```python
from build123d import *

# Parameters (mm, degrees)
ESBO_O1_W                = 86.5
ESBO_O1_H                = 54.64
RESSALTO_EXTRUS_O2_DEPTH = 2
ESBO_O3_R                = 1.59
CORTE_EXTRUS_O1_DEPTH    = 2
FILETE1_R                = 12
FILETE2_R                = 12
ESBO_O4_R                = 5
ESBO_O4_R_2              = 4
ESBO_O4_W                = 6
ESBO_O4_H                = 8.5
CORTE_EXTRUS_O2_DEPTH    = 10


with BuildPart() as part:
    # Esboço1 → Ressalto-extrusão2 (new body)
    with BuildSketch(Plane.XY):
        with Locations((43.25, 27.32)):
            Rectangle(ESBO_O1_W, ESBO_O1_H)
    extrude(amount=RESSALTO_EXTRUS_O2_DEPTH)

    # Esboço3 → Corte-extrusão1 (cut)
    with BuildSketch(Plane(origin=(0, 0, 0), x_dir=(-1, 0, 0), z_dir=(0, 0, -1))):
        with Locations((-71.89, 51.46)):
            Circle(ESBO_O3_R)
        with Locations((-71.89, 3.18)):
            Circle(ESBO_O3_R)
        with Locations((-5.72, 6.35)):
            Circle(ESBO_O3_R)
        with Locations((-5.72, 48.29)):
            Circle(ESBO_O3_R)
    extrude(amount=-CORTE_EXTRUS_O1_DEPTH, mode=Mode.SUBTRACT)

    # Filete1
    filete1_edges = [part.edges().sort_by_distance(p)[0] for p in [
        (0, 54.64, 1),
    ]]
    fillet(filete1_edges, radius=FILETE1_R)

    # Filete2
    filete2_edges = [part.edges().sort_by_distance(p)[0] for p in [
        (0, 0, 1),
    ]]
    fillet(filete2_edges, radius=FILETE2_R)

    # Esboço4 → Corte-extrusão2 (cut)
    with BuildSketch(Plane.XY.offset(2)):
        with Locations((24.86, 48.58)):
            Circle(ESBO_O4_R)
        with Locations((39.09, 49.5)):
            Circle(ESBO_O4_R_2)
        with Locations((64.16, 46.97)):
            Circle(ESBO_O4_R_2)
        with Locations((83.5, 38.39)):
            Rectangle(ESBO_O4_W, ESBO_O4_H)
    extrude(amount=-CORTE_EXTRUS_O2_DEPTH, mode=Mode.SUBTRACT)


solid = part.part
```
Source: CAD feature listing. Evaluate the final solid. Frame: model axes, mm. A direction names the side the tool comes from. Coordinates: 2 decimals unless noted, no trailing zeros. Write each loop counter-clockwise with the first axis right and the second up, starting at its lowest first coordinate (ties: lowest second). Pieces come first, ordered by that corner, then holes. Notation, with made-up numbers: (3, -16.5) -> (23, -16.5) arc R36 cw to (23, 22.5) -> close; hole circle Ø1 at (73.5, 60.5). An arc over 180 degrees is marked (long way). Return JSON: item names as keys, results as strings. Group by question number.
1) Contact query for a flat-ended pin moving along its axis: P1, Ø5, axis at x = 64.16, y = 46.97, coming from the -Z side. Output: stop coordinate, or through.
2) Section query B-B, the plane x = 24.86. Return loops of the section in (y, z).
3) Section query C-C, the plane z = 1.3. Return loops of the section in (x, y).
4) Ray query, line 1 along Y through (x, z) = (71.89, 0.65); line 2 along Y through (x, z) = (39.09, 1.3); line 3 along Y through (x, z) = (5.72, 0.7). Return the intervals inside material, ascending.
5) Section query A-A, the plane x = 71.89. Return loops of the section in (y, z), plus the area to 3 significant figures.
6) Set-up query: faces 5 (the face through (80.5, 38, 1)), 6 (the face through (49, 0, 1)). Return all of +Z, -Z, +X, -X, +Y, -Y with unobstructed straight access to the full face (end or side cutting, diameter ignored); none if empty.
7) Section query D-D, the plane y = 6.35. Return loops of the section in (x, z), plus the area to 3 significant figures.
8) Mould query, pull axis Y, two halves, no side actions, for faces 1 (the face through (3.42, 51.03, 1.01)), 2 (the face through (83, 42.64, 1)), 3 (the face through (0, 27, 1)), 4 (the face through (3.42, 3.61, 1.01)). Classes: +Y half, -Y half, draft (parallel to the pull), parting line (faces both ways), or undercut.
From the geometry:
{
 "1": {"P1": "through"},
 "2": {"outline": "(0, 0) -> (43.58, 0) -> (43.58, 2) -> (0, 2) -> close; (53.58, 0) -> (54.64, 0) -> (54.64, 2) -> (53.58, 2) -> close"},
 "3": {"outline": "(0, 12) arc R12 ccw to (12, 0) -> (86.5, 0) -> (86.5, 34.14) -> (80.5, 34.14) -> (80.5, 42.64) -> (86.5, 42.64) -> (86.5, 54.64) -> (12, 54.64) arc R12 ccw to (0, 42.64) -> close; hole circle Ø3.18 at (5.72, 6.35); hole circle Ø3.18 at (5.72, 48.29); hole circle Ø10 at (24.86, 48.58); hole circle Ø8 at (39.09, 49.5); hole circle Ø8 at (64.16, 46.97); hole circle Ø3.18 at (71.89, 3.18); hole circle Ø3.18 at (71.89, 51.46)"},
 "4": {"line 1": "0 to 1.59, 4.77 to 49.87, 53.05 to 54.64", "line 2": "0 to 45.5, 53.5 to 54.64", "line 3": "1.77 to 4.76, 7.94 to 46.7, 49.88 to 52.87"},
 "5": {"outline": "(0, 0) -> (1.59, 0) -> (1.59, 2) -> (0, 2) -> close; (4.77, 0) -> (49.87, 0) -> (49.87, 2) -> (4.77, 2) -> close; (53.05, 0) -> (54.64, 0) -> (54.64, 2) -> (53.05, 2) -> close", "area": "96.6 mm²"},
 "6": {"face 5": "+Z, -Z, +X", "face 6": "+Z, -Z, +X, -X, -Y"},
 "7": {"outline": "(1.41, 0) -> (4.13, 0) -> (4.13, 2) -> (1.41, 2) -> close; (7.31, 0) -> (86.5, 0) -> (86.5, 2) -> (7.31, 2) -> close", "area": "164 mm²"},
 "8": {"face 1": "+Y half", "face 2": "undercut", "face 3": "draft", "face 4": "-Y half"}
}
